Answer from the drawing. Dimensions are ordinates in mm from the lowest x, y and z of the part. A direction names the side the tool comes from. Give positions to 0.01 mm unless a question says otherwise; leave off trailing zeros. Order: outer loops, then holes, each group sorted by start corner. A loop starts at its lowest first (then second) coordinate and runs counter-clockwise, first axis right, second up. Notation, with made-up numbers: M 77,87.25 L 127,87.25 A15 ccw 127,97.25 Z; hole C 2.25,-4 d8. An arc over 180 degrees is marked long. One line per item, written item: value.
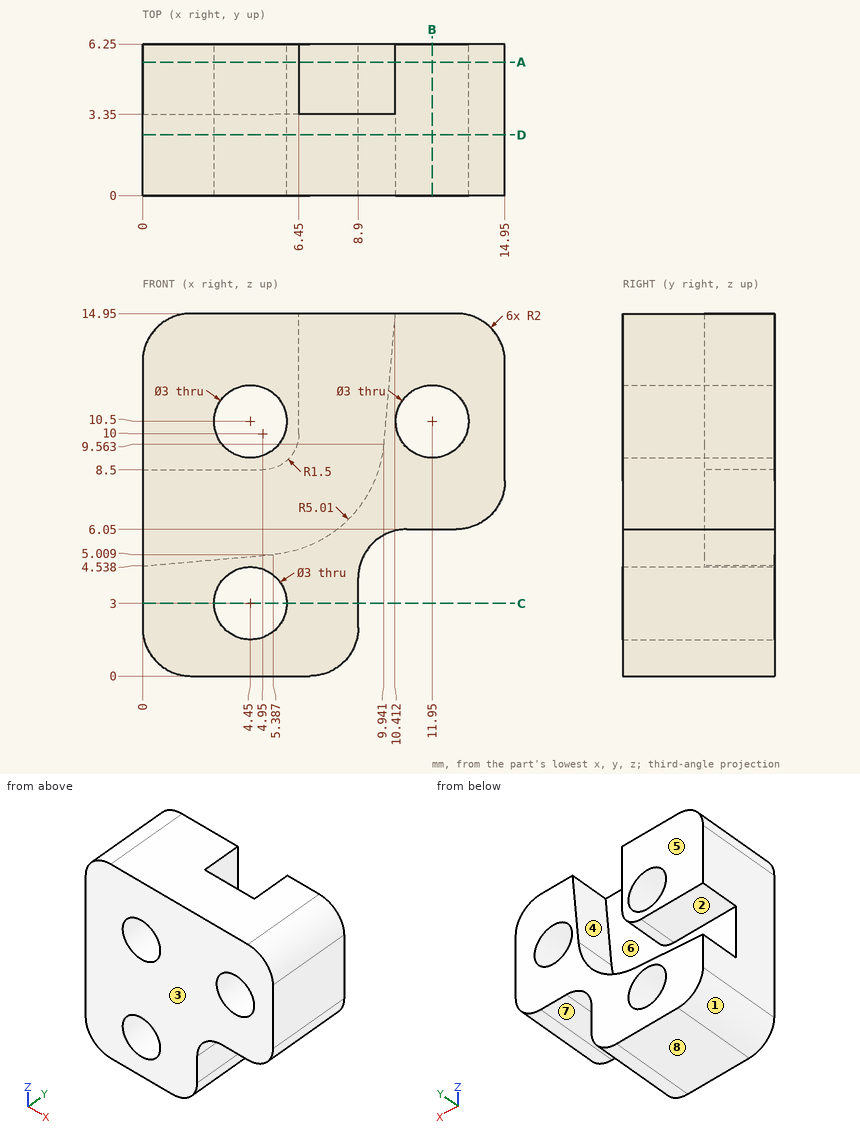
(1) Section C-C, the plane z = 3 is taken. Give the vertices of the cut face in (x, y).
Findings:
outline: M 0,0 L 2.95,0 L 2.95,6.25 L 0,6.25 Z; M 5.95,0 L 8.9,0 L 8.9,6.25 L 5.95,6.25 Z
(2) Section D-D, the plane y = 2.5 is taken. Give the vertices of the cut face in (x, z).
Findings:
outline: M 0,2 A2 ccw 2,0 L 6.9,0 A2 ccw 8.9,2 L 8.9,4.05 A2 cw 10.9,6.05 L 12.95,6.05 A2 ccw 14.95,8.05 L 14.95,12.95 A2 ccw 12.95,14.95 L 2,14.95 A2 ccw 0,12.95 Z; hole C 4.45,3 d3; hole C 4.45,10.5 d3; hole C 11.95,10.5 d3
(3) Find the intervals of material crossed by probe 1 along X at (y, z) = (1.5, 10.5); probe 2 along X at (y, z) = (2.5, 3); probe 3 along Y at (x, z) = (8.25, 7), in increasing order. Write a range as from..to.
Findings:
probe 1: x = 0..2.95, 5.95..10.45, 13.45..14.95
probe 2: x = 0..2.95, 5.95..8.9
probe 3: y = 0..3.35
(4) Which of the six approach directions +Z, -Z, +X, -X, +Y, -Y give full straight-line access (tool end or side, diameter ignored) to the marked faces 4, 5, 6, 7 and 8?
Findings:
face 4: +Z, +Y
face 5: +Z, -Z, +X, -X, +Y
face 6: +Y
face 7: -Z, +X, +Y, -Y
face 8: -Z, +X, -X, +Y, -Y
(5) Given P1, Ø2.5, axis at x = 11.95, z = 10.5, coming from the +Y side; P2, Ø2.5, axis at y = 2.5, z = 2.5, coming from the +X side; P3, Ø1.6, axis at x = 12, y = 4, coming from the -Z side, each flat-ended and moving along its own axis, determine where each tip first touches the part or whether it passes through.
Findings:
P1: passes through
P2: stops at x = 8.9
P3: stops at z = 6.05
(6) Determine the mould class of the marked faces 1, 2 and 3 for opening direction Z: pulls with the +Z half, pulls with the -Z half, needs draft (parallel to the pull), parting line crosses it, or undercut.
Findings:
face 1: pulls with the -Z half
face 2: undercut
face 3: needs draft
(7) Section A-A, the plane y = 5.5 is taken. Give the vertices of the cut face in (x, z).
Findings:
outline: M 0,2 A2 ccw 2,0 L 6.9,0 A2 ccw 8.9,2 L 8.9,4.05 A2 cw 10.9,6.05 L 12.95,6.05 A2 ccw 14.95,8.05 L 14.95,12.95 A2 ccw 12.95,14.95 L 10.41,14.95 L 9.94,9.56 A5.01 cw 5.39,5.01 L 0,4.54 Z; M 0,8.5 L 4.95,8.5 A1.5 ccw 6.45,10 L 6.45,14.95 L 2,14.95 A2 ccw 0,12.95 Z; hole C 4.45,3 d3; hole C 4.45,10.5 d3; hole C 11.95,10.5 d3
(8) Section B-B, the plane x = 11.95 is taken. Give the vertices of the cut face in (y, z), then the cut area to 3 significant figures.
Findings:
outline: M 0,6.05 L 6.25,6.05 L 6.25,9 L 0,9 Z; M 0,12 L 6.25,12 L 6.25,14.95 L 0,14.95 Z
area: 36.9 mm^2
